Study the drawing (mm; zero at the part's minimum x, y, z) and answer. A direction names the side the tool comes from. Round coordinates to 2 decimals unless told otherwise and drop trailing zeros. Loops run counter-clockwise (first coordinate to the right, second up) from the corner with the lowest first, then second, coordinate; pieces in that order, holes last. Notation, with made-up numbers: M 12,-17 L 46,-17 A25 ccw 46,-2 Z; hole C 49.5,65 d3. An arc over 180 degrees is marked long. Put each result on its own line as item: value. Start each with the question number.
(1) Which of the six approach directions +Z, -Z, +X, -X, +Y, -Y give full straight-line access (tool end or side, diameter ignored) to the marked faces 1, 2 and 3?
(2) Section D-D, the plane x = 7 is taken. Determine the outline of the cut face in (y, z).
(3) Section A-A, the plane y = 7 is taken. Determine the outline of the cut face in (x, z), then the cut area to 3 significant figures.
(4) Flat-ended cylindrical pins translate along their axes: P1, Ø1.5, axis at x = 52.5, z = 11, coming from the +Y side; P2, Ø3, axis at x = 69.5, z = 12, coming from the -Y side; P3, Ø1, axis at x = 9, z = 5, coming from the +Y side. Find the tip coordinate at first contact, or state that the pin passes through.
(5) Straight lines are drawn through the part: line 1 (Z direction, x = 39.5, y = 7.25); line 2 (X direction, y = 13.5, z = 7). For each, find the intervals that lie inside material, in ascending order.
(6) Section C-C, the plane x = 66.5 is taken. Determine the outline of the cut face in (y, z), then the cut area to 3 significant figures.
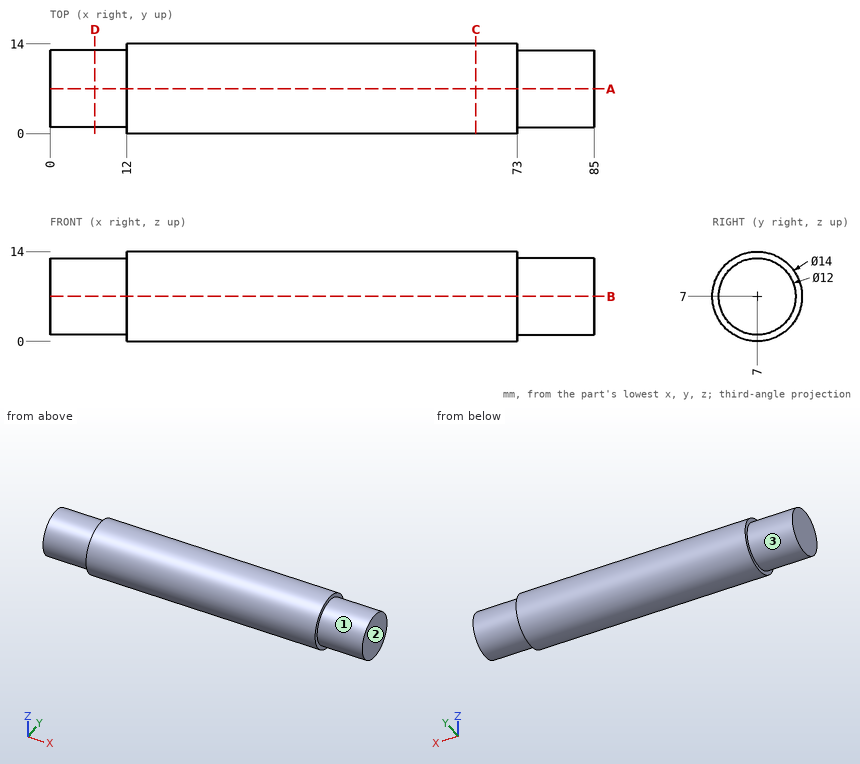
Recorded:
1. face 1: +X
1. face 2: +Z, -Z, +X, +Y, -Y
1. face 3: -X
2. outline: C 7,7 d12
3. outline: M 0,1 L 12,1 L 12,0 L 73,0 L 73,1 L 85,1 L 85,13 L 73,13 L 73,14 L 12,14 L 12,13 L 0,13 Z
3. area: 1,140 mm²
4. P1: stops at y = 13.2
4. P2: stops at y = 0.94
4. P3: stops at y = 12.81
5. line 1: z = 0 to 14
5. line 2: x = 12 to 73
6. outline: C 7,7 d14
6. area: 154 mm²
